Geometry: final body of the model. Coordinates: model frame, mm. A direction names the side the tool comes from. Round coordinates to 2 decimals unless told otherwise and drop trailing zeros. Loops run counter-clockwise (first coordinate to the right, second up) from the corner with the lowest first, then second, coordinate; pieces in that order, holes last. Notation, with made-up numbers: (81.25, 76.5) - (112.25, 76.5) arc R17 cw to (112.25, 81.5) - close; hole circle Ø2 at (48, 56.25). An arc over 180 degrees is marked (long way). Write item = value, one per line. Start each with the question number.
Item 1: Access query for faces 1 (the flat face through (-15, -113, 18)), 2 (the flat face through (0, -98.7, -18)). Directions: +Z, -Z, +X, -X, +Y, -Y. A direction counts if a zero-diameter tool reaches every point of the face in a straight line with its end or side. Return the directions, or none.
Item 2: Section C-C (z = -18). Count the separate pieces of the cut face and the enclosed holes in it, plus the area to 3 significant figures.
Item 3: Line query: line 1 (X direction, y = -71.5, z = 17); line 2 (X direction, y = -101, z = -12). Output: solid intervals per line, ascending. Write a range as from..to.
Item 4: Section A-A (z = -1). Return loops of the section in (x, y).
Item 5: Section B-B (y = -131.5). Return loops of the section in (x, z).
Item 6: Section D-D (y = -48). Return loops of the section in (x, z).
from build123d import *

# Parameters (mm, degrees)
F0_W      = 48
F0_H      = 48
F0_W_2    = 40.2
F0_H_2    = 40.2
F1_DEPTH  = 150
F2_W      = 30
F2_H      = 5
F3_DEPTH  = 2.7
F5_W      = 30
F5_H      = 5
F6_DEPTH  = 9
F8_W      = 30
F8_H      = 5
F9_DEPTH  = 9
F11_W     = 30
F11_H     = 5
F12_DEPTH = 9
F14_W     = 30
F14_H     = 5
F15_DEPTH = 9
F17_W     = 30
F17_H     = 5
F18_DEPTH = 9
F20_W     = 30
F20_H     = 5
F21_DEPTH = 9
F23_W     = 30
F23_H     = 5
F24_DEPTH = 9
F26_W     = 30
F26_H     = 5
F27_DEPTH = 2.7


with BuildPart() as f1:
    # F0 (on Front) → F1 (new body)
    with BuildSketch(Plane.XZ):
        Rectangle(F0_W, F0_H)
        Rectangle(F0_W_2, F0_H_2, mode=Mode.SUBTRACT)
    extrude(amount=F1_DEPTH)

    # F2 (on Front) → F3 (join)
    with BuildSketch(Plane.XZ):
        with Locations((0, 17.6)):
            Rectangle(F2_W, F2_H)
        with Locations((0, -17.6)):
            Rectangle(F2_W, F2_H)
    extrude(amount=F3_DEPTH)

    # F5 (on offset) → F6 (join)
    with BuildSketch(Plane.XZ.offset(12.9)):
        with Locations((0, 17.601031)):
            Rectangle(F5_W, F5_H)
        with Locations((0, -17.6)):
            Rectangle(F5_W, F5_H)
    extrude(amount=F6_DEPTH)

    # F8 (on offset) → F9 (join)
    with BuildSketch(Plane.XZ.offset(32.1)):
        with Locations((0, 17.6)):
            Rectangle(F8_W, F8_H)
        with Locations((0, -17.6)):
            Rectangle(F8_W, F8_H)
    extrude(amount=F9_DEPTH)

    # F11 (on offset) → F12 (join)
    with BuildSketch(Plane.XZ.offset(51.3)):
        with Locations((0, -17.6)):
            Rectangle(F11_W, F11_H)
        with Locations((0, 17.6)):
            Rectangle(F11_W, F11_H)
    extrude(amount=F12_DEPTH)

    # F14 (on offset) → F15 (join)
    with BuildSketch(Plane.XZ.offset(70.5)):
        with Locations((0, 17.6)):
            Rectangle(F14_W, F14_H)
        with Locations((0, -17.6)):
            Rectangle(F14_W, F14_H)
    extrude(amount=F15_DEPTH)

    # F17 (on offset) → F18 (join)
    with BuildSketch(Plane.XZ.offset(89.7)):
        with Locations((0, 17.6)):
            Rectangle(F17_W, F17_H)
        with Locations((0, -17.6)):
            Rectangle(F17_W, F17_H)
    extrude(amount=F18_DEPTH)

    # F20 (on offset) → F21 (join)
    with BuildSketch(Plane.XZ.offset(108.9)):
        with Locations((0, 17.6)):
            Rectangle(F20_W, F20_H)
        with Locations((0, -17.6)):
            Rectangle(F20_W, F20_H)
    extrude(amount=F21_DEPTH)

    # F23 (on offset) → F24 (join)
    with BuildSketch(Plane.XZ.offset(128.1)):
        with Locations((0, 17.6)):
            Rectangle(F23_W, F23_H)
        with Locations((0, -17.6)):
            Rectangle(F23_W, F23_H)
    extrude(amount=F24_DEPTH)

    # F26 (on offset) → F27 (join)
    with BuildSketch(Plane.XZ.offset(147.3)):
        with Locations((0, 17.6)):
            Rectangle(F26_W, F26_H)
        with Locations((0, -17.6)):
            Rectangle(F26_W, F26_H)
    extrude(amount=F27_DEPTH)


solid = f1.part
Taken from the geometry:
q1.face_1 = +Y, -Y
q1.face_2 = none
q2.separate_pieces = 11
q2.enclosed_holes = 0
q2.area = 3,220 mm^2
q3.line_1 = -24..-20.1, -15..15, 20.1..24
q3.line_2 = -24..-20.1, 20.1..24
q4.outline = (-24, -150) - (-20.1, -150) - (-20.1, 0) - (-24, 0) - close; (20.1, -150) - (24, -150) - (24, 0) - (20.1, 0) - close
q5.outline = (-24, -24) - (24, -24) - (24, 24) - (-24, 24) - close; hole (-20.1, -20.1) - (-15, -20.1) - (-15, -15.1) - (15, -15.1) - (15, -20.1) - (20.1, -20.1) - (20.1, 20.1) - (15, 20.1) - (15, 15.1) - (-15, 15.1) - (-15, 20.1) - (-20.1, 20.1) - close
q6.outline = (-24, -24) - (24, -24) - (24, 24) - (-24, 24) - close; hole (-20.1, -20.1) - (20.1, -20.1) - (20.1, 20.1) - (-20.1, 20.1) - close
